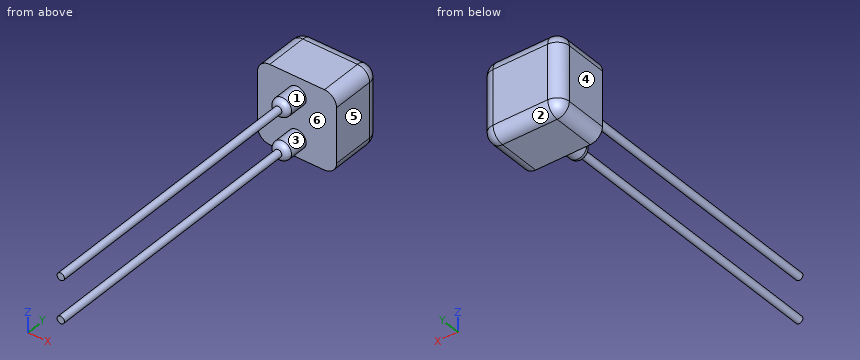
Autodesk Inventor part; units mm, degrees
ref_plane "YZ Plane" through (0, 0, 0) normal (1, 0, 0) x (0, 1, 0)
ref_plane "XZ Plane" through (0, 0, 0) normal (0, 1, 0) x (-1, 0, 0)
ref_plane "XY Plane" through (0, 0, 0) normal (0, 0, 1) x (1, 0, 0)
sketch "Sketch1" plane through (0, 0, 0) normal (0, 1, 0) x (-1, 0, 0)
  line L0 (1, 0) -> (5.5, 0)
  line L1 (6.5, -1) -> (6.5, -5.5)
  line L2 (5.5, -6.5) -> (1, -6.5)
  line L3 (0, -5.5) -> (0, -1)
  arc A0 (6.5, -1) -> (5.5, 0) centre (5.5, -1) ccw
  arc A1 (0, -5.5) -> (1, -6.5) centre (1, -5.5) ccw
  arc A2 (5.5, -6.5) -> (6.5, -5.5) centre (5.5, -5.5) ccw
  arc A3 (1, 0) -> (0, -1) centre (1, -1) ccw
  circle A4 centre (3.25, -5) radius 0.75
  circle A5 centre (3.25, -1.5) radius 0.75
  point P0 (0, 0)
  point P1 (6.5, -6.5)
  point P2 (6.5, 0)
  point P3 (0, -6.5)
  dimension "d0" = 6.5
  dimension "d1" = 6.5
  dimension "d2" = 1
  dimension "d5" = 1.5
  dimension "d7" = 1.5
extrude "Extrusion1" add sketch "Sketch1" along normal blind 4.5 contours L0 A0 L1 A2 L2 A1 L3 A3 | A4 | A5
fillet "Fillet1" radius 1 8 edges at (-0.2929, 4.5, -6.2071) (-3.25, 4.5, -6.5) (-6.2071, 4.5, -6.2071) (-6.5, 4.5, -3.25) (-6.2071, 4.5, -0.2929) (-3.25, 4.5, 0) (-0.2929, 4.5, -0.2929) (0, 4.5, -3.25)
sketch "Sketch2" plane through (0, 0, 0) normal (0, -1, 0) x (1, 0, 0)
  circle A0 centre (-3.25, -1.5) radius 0.75
  circle A1 centre (-3.25, -5) radius 0.75
  point P0 (0, 0)
  dimension "d13" = 1.5
  dimension "d14" = 1.5
extrude "Extrusion2" add sketch "Sketch2" along normal blind 2
sketch "Sketch3" plane through (-3.25, -2, -1.5) normal (0, -1, 0) x (1, 0, 0)
  circle A0 centre (0, 0) radius 0.3
  circle A1 centre (0, -3.5) radius 0.75
  circle A2 centre (0, -3.5) radius 0.3
  point P0 (3.25, 1.5)
  dimension "d17" = 0.6
  dimension "d18" = 0.6
extrude "Extrusion3" add sketch "Sketch3" along normal blind 23 contours A0 | A2
fillet "Fillet2" radius 0.45 2 edges at (-4, -2, -1.5) (-4, -2, -5)
equation "\"BendRadius\" = Thickness"
equation "\"BendReliefWidth\" = Thickness"
equation "\"BendReliefDepth\" = 0.5 * Thickness"
equation "\"CornerReliefSize\" = 4 * Thickness"
equation "\"MinimumRemnant\" = 2 * Thickness"
equation "\"TransitionRadius\" = BendRadius"
equation "\"JacobiRadiusSize\" = BendRadius"
equation "\"GapSize\" = Thickness"
Verification items for the finished model (mm, model axes). Face numbers are marked on the shaded views. A direction names the side the tool comes from. Coordinates: 2 decimals unless noted, no trailing zeros. Write each loop counter-clockwise with the first axis right and the second up, starting at its lowest first coordinate (ties: lowest second). Pieces come first, ordered by that corner, then holes. Notation, with made-up numbers: M 67.25,12 L 114.25,12 A27 cw 114.25,30 Z; hole C -39.75,-6.75 d1. An arc over 180 degrees is marked long. One line per item, written item: value.
Item 1: Scan lines: line 1 along Y through (x, z) = (-1.25, -4.5); line 2 along Z through (x, y) = (-3.5, -17.75); line 3 along X through (y, z) = (-21.75, -1.75). Record each from-to range of solid material in increasing order.
Check sheet entries:
line 1: y = 0 to 4.5
line 2: z = -5.17 to -4.83, -1.67 to -1.33
line 3: x = -3.42 to -3.08
Item 2: Section check B-B, the plane x = -4.25. Record the boundary of the cut face in (y, z).
Check sheet entries:
outline: M 0,-6.5 L 3.5,-6.5 A1 ccw 4.5,-5.5 L 4.5,-1 A1 ccw 3.5,0 L 0,0 Z
Item 3: Section check C-C, the plane y = -1. Record the boundary of the cut face in (x, z).
Check sheet entries:
outline: C -3.25,-5 d1.5; C -3.25,-1.5 d1.5
Item 4: Gauge pin test, flat ends, axial feed: pin 1 Ø2 at (x, z) = (-0.5, -4) entering from -Y; pin 2 Ø1.5 at (y, z) = (-21.5, -5.5) entering from -X. Record the tip position at first contact, or that the pin passes through.
Check sheet entries:
pin 1: stops at y = 0
pin 2: stops at x = -3.55
Item 5: Section check A-A, the plane y = -13.5. Record the boundary of the cut face in (x, z), plus the area to 3 significant figures.
Check sheet entries:
outline: C -3.25,-5 d0.6; C -3.25,-1.5 d0.6
area: 0.565 mm^2
Item 6: Mould release check, pull along Z, two halves, no side actions. Record for the marked faces 1, 2, 3 and 4: pulls with the +Z half, pulls with the -Z half, needs draft (parallel to the pull), parting line crosses it, or undercut.
Check sheet entries:
face 1: undercut
face 2: pulls with the -Z half
face 3: undercut
face 4: needs draft
Item 7: Access from +Z, -Z, +X, -X, +Y, -Y to the whole of each face (thin tool, end or side, straight path). Record for the marked faces 5 and 6.
Check sheet entries:
face 5: +Z, -Z, +X, +Y, -Y
face 6: -Y
Item 8: Section check D-D, the plane z = -0.25. Record the boundary of the cut face in (x, y), plus the area to 3 significant figures.
Check sheet entries:
outline: M -6.16,0 L -0.34,0 L -0.34,3.5 A0.66 ccw -1,4.16 L -5.5,4.16 A0.66 ccw -6.16,3.5 Z
area: 24.0 mm^2
